from build123d import *

# Parameters (mm, degrees)
F0_W      = 406.4
F0_H      = 76.2
F1_DEPTH  = 6.35
F2_W      = 50.8
F2_H      = 25.4
F3_DEPTH  = 6.35
F4_W      = 50.8
F4_H      = 25.4
F5_DEPTH  = 6.35
F7_W      = 38.1
F7_H      = 6.35
F6_W      = 38.1
F6_H      = 6.35
F8_DEPTH  = 88.901
F10_DEPTH = 6.35
F12_D     = 12.7


with BuildPart() as f1:
    # F0 (on Top) → F1 (new body)
    with BuildSketch(Plane.XY):
        Rectangle(F0_W, F0_H)
    extrude(amount=F1_DEPTH)

    # F2 (on face) → F3 (join)
    with BuildSketch(Plane.XZ.offset(38.1)):
        with Locations((76.2, -6.35)):
            Rectangle(F2_W, F2_H)
        with Locations((-76.2, -6.35)):
            Rectangle(F2_W, F2_H)
    extrude(amount=F3_DEPTH)

    # F4 (on face) → F5 (join)
    with BuildSketch(Plane(origin=(0, 38.1, 0), x_dir=(-1, 0, 0), z_dir=(0, 1, 0))):
        with Locations((-76.2, -6.35)):
            Rectangle(F4_W, F4_H)
        with Locations((76.2, -6.35)):
            Rectangle(F4_W, F4_H)
    extrude(amount=F5_DEPTH)

    # F7 (on face) + F6 (on face) → F8 (cut, through all)
    with BuildSketch(Plane(origin=(0, 44.45, 0), x_dir=(-1, 0, 0), z_dir=(0, 1, 0))):
        with Locations((76.2, -9.525)):
            Rectangle(F7_W, F7_H)
    with BuildSketch(Plane(origin=(0, 44.45, 0), x_dir=(-1, 0, 0), z_dir=(0, 1, 0))):
        with Locations((-76.2, -9.525)):
            Rectangle(F6_W, F6_H)
    extrude(amount=-F8_DEPTH, mode=Mode.SUBTRACT)

    # F9 (on face) → F10 (join)
    with BuildSketch(Plane.XY.offset(6.35)):
        Polygon((-101.6, 38.1), (-203.2, 38.1), (-203.2, -38.1), (-101.6, -38.1), (-101.6, -44.45), (-50.8, -44.45), (-50.8, -38.1), (50.8, -38.1), (50.8, -44.45), (101.6, -44.45), (101.6, -38.1), (203.2, -38.1), (203.2, 38.1), (101.6, 38.1), (101.6, 44.45), (50.8, 44.45), (50.8, 38.1), (-50.8, 38.1), (-50.8, 44.45), (-101.6, 44.45), align=None)
    extrude(amount=F10_DEPTH)

    # F12 (through all)
    with Locations(Plane.XY.offset(12.7)):
        with Locations((177.8, 0), (-76.2, 0)):
            Hole(F12_D / 2)


solid = f1.part
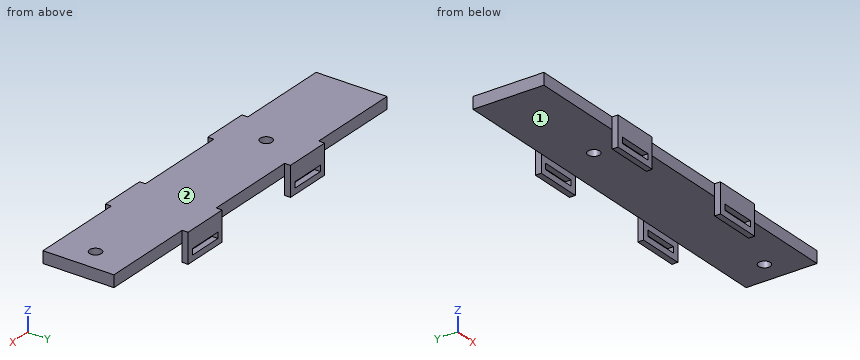
Design review of the part built by this model. Coordinates are the model's own, in mm. Face numbers are marked on the shaded views. Give positions to 0.01 mm unless a question says otherwise; leave off trailing zeros. Loops run counter-clockwise (first coordinate to the right, second up) from the corner with the lowest first, then second, coordinate; pieces in that order, holes last. Notation, with made-up numbers: (70, 54) -> (121, 54) arc R25 ccw to (121, 81) -> close; hole circle Ø7 at (12, -33). An arc over 180 degrees is marked (long way). One line per question, with ' | ' between items. Start each with the question number.
(1) We need section C-C (z = 6.5). State the section outline as (x, y) points.
(2) Insertion check: P1, Ø3, axis at y = -40, z = -8.5, coming from the -X side; P2, Ø12, axis at x = -45.5, z = -13.5, coming from the +Y side; P3, Ø14, axis at x = 140.5, z = 5.5, coming from the -Y side; P4, Ø3, axis at y = -42.5, z = -2.5, coming from the +X side. Each pin has a flat end and moves straight along its axis. Give the tip position at first contact, or say it passes through.
(3) We need section B-B (y = 0). State the section outline as (x, z) points.
(4) Draft analysis for pull direction Y (two halves, no side actions). For the marked faces 1 and 2, state which applies: +Y half, -Y half, draft (parallel to the pull), parting line (faces both ways), or undercut.
(5) We need section D-D (x = -76.2). State the section outline as (y, z) points, and give its area (3 significant figures).
(6) For line 1 (Y direction, x = -60, z = -1); line 2 (Y direction, x = -76, z = 8); line 3 (Z direction, x = 181.5, y = -30.5), list the stretches that pass through material, from the lowest coordinate up.
(7) We need section A-A (x = 177.8). State the section outline as (y, z) points, and give its area (3 significant figures).
The answers:
1) outline: (-203.2, -38.1) -> (-101.6, -38.1) -> (-101.6, -44.45) -> (-50.8, -44.45) -> (-50.8, -38.1) -> (50.8, -38.1) -> (50.8, -44.45) -> (101.6, -44.45) -> (101.6, -38.1) -> (203.2, -38.1) -> (203.2, 38.1) -> (101.6, 38.1) -> (101.6, 44.45) -> (50.8, 44.45) -> (50.8, 38.1) -> (-50.8, 38.1) -> (-50.8, 44.45) -> (-101.6, 44.45) -> (-101.6, 38.1) -> (-203.2, 38.1) -> close; hole circle Ø12.7 at (-76.2, 0); hole circle Ø12.7 at (177.8, 0)
2) P1: stops at x = -101.6 | P2: stops at y = 44.45 | P3: stops at y = -38.1 | P4: stops at x = 101.6
3) outline: (-203.2, 0) -> (-82.55, 0) -> (-82.55, 12.7) -> (-203.2, 12.7) -> close; (-69.85, 0) -> (171.45, 0) -> (171.45, 12.7) -> (-69.85, 12.7) -> close; (184.15, 0) -> (203.2, 0) -> (203.2, 12.7) -> (184.15, 12.7) -> close
4) face 1: undercut | face 2: draft
5) outline: (-44.45, -19.05) -> (-38.1, -19.05) -> (-38.1, -12.7) -> (-44.45, -12.7) -> close; (-44.45, -6.35) -> (-38.1, -6.35) -> (-38.1, 0) -> (-6.35, 0) -> (-6.35, 12.7) -> (-44.45, 12.7) -> close; (6.35, 0) -> (38.1, 0) -> (38.1, -6.35) -> (44.45, -6.35) -> (44.45, 12.7) -> (6.35, 12.7) -> close; (38.1, -19.05) -> (44.45, -19.05) -> (44.45, -12.7) -> (38.1, -12.7) -> close | area: 1,130 mm^2
6) line 1: y = -44.45 to -38.1, 38.1 to 44.45 | line 2: y = -44.45 to -6.35, 6.35 to 44.45 | line 3: z = 0 to 12.7
7) outline: (-38.1, 0) -> (-6.35, 0) -> (-6.35, 12.7) -> (-38.1, 12.7) -> close; (6.35, 0) -> (38.1, 0) -> (38.1, 12.7) -> (6.35, 12.7) -> close | area: 806 mm^2
